The figure shows three views and two pictorial views of one solid part (mm, origin at its lowest corner). Answer the questions. Give positions to 0.01 mm unless a question says otherwise; leave off trailing zeros. Write each loop counter-clockwise with the first axis right and the second up, starting at its lowest first coordinate (ties: lowest second). Pieces come first, ordered by that corner, then holes. Notation, with made-up numbers: (43.5, 3.5) -> (51.5, 3.5) arc R37 cw to (51.5, 42.5) -> close; hole circle Ø6 at (-5.5, 17.5). An arc over 180 degrees is marked (long way). Write item = value, one per line. Start each with the question number.
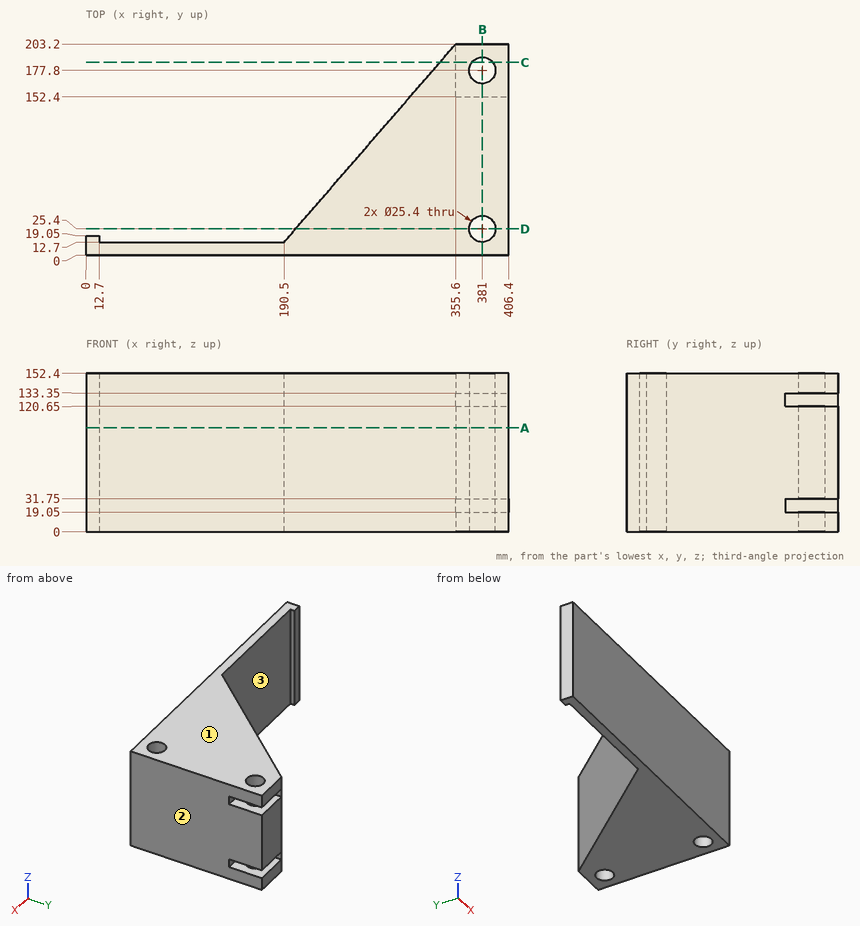
(1) A cutting plane is placed at A-A, the plane z = 100. Write down the section's boundary in (x, y).
(2) Find the intervals of material crossed by line 1 along Y through (x, z) = (380, 44); line 2 along X through (y, z) = (177, 148); line 3 along Y through (x, z) = (20.5, 17), in increasing order.
(3) A cutting plane is placed at D-D, the plane y = 25.4. Write down the section's boundary in (x, z), then the cut area to 3 significant figures.
(4) A cutting plane is placed at B-B, the plane x = 381. Write down the section's boundary in (y, z).
(5) Determine the mould class of the marked faces 1, 2 and 3 for opening direction X: pulls with the +X half, pulls with the -X half, needs draft (parallel to the pull), parting line crosses it, or undercut.
(6) Each of these flat-tipped pins is pushed along its axis until it touches: pin 1 (14 mm diameter, centred on y = 178.5, z = 24, fed in from +X); pin 2 (1 mm diameter, centred on y = 169, z = 124.5, fed in from -X); pin 3 (6.5 mm diameter, centred on x = 4, z = 80, fed in from +Y); pin 4 (1.5 mm diameter, centred on x = 211.5, z = 77, fed in from +Y). Where does it stop, or does it pass through?
(7) A cutting plane is placed at C-C, the plane y = 185.5. Write down the section's boundary in (x, z), then the cut area to 3 significant figures.
Results list:
q1.outline = (0, 0) -> (406.4, 0) -> (406.4, 203.2) -> (355.6, 203.2) -> (190.5, 12.7) -> (12.7, 12.7) -> (12.7, 19.05) -> (0, 19.05) -> close; hole circle Ø25.4 at (381, 25.4); hole circle Ø25.4 at (381, 177.8)
q2.line_1 = 0 to 12.74, 38.06 to 165.14, 190.46 to 203.2
q2.line_2 = 332.89 to 368.33, 393.67 to 406.4
q2.line_3 = 0 to 12.7
q3.outline = (201.51, 0) -> (368.3, 0) -> (368.3, 152.4) -> (201.51, 152.4) -> close; (393.7, 0) -> (406.4, 0) -> (406.4, 152.4) -> (393.7, 152.4) -> close
q3.area = 27,400 mm²
q4.outline = (0, 0) -> (12.7, 0) -> (12.7, 152.4) -> (0, 152.4) -> close; (38.1, 0) -> (165.1, 0) -> (165.1, 19.05) -> (152.4, 19.05) -> (152.4, 31.75) -> (165.1, 31.75) -> (165.1, 120.65) -> (152.4, 120.65) -> (152.4, 133.35) -> (165.1, 133.35) -> (165.1, 152.4) -> (38.1, 152.4) -> close; (190.5, 0) -> (203.2, 0) -> (203.2, 19.05) -> (190.5, 19.05) -> close; (190.5, 31.75) -> (203.2, 31.75) -> (203.2, 120.65) -> (190.5, 120.65) -> close; (190.5, 133.35) -> (203.2, 133.35) -> (203.2, 152.4) -> (190.5, 152.4) -> close
q5.face_1 = needs draft
q5.face_2 = pulls with the +X half
q5.face_3 = undercut
q6.pin_1 = 406.4
q6.pin_2 = 325.53
q6.pin_3 = 19.05
q6.pin_4 = 37.8
q7.outline = (340.26, 0) -> (370.9, 0) -> (370.9, 19.05) -> (355.6, 19.05) -> (355.6, 31.75) -> (370.9, 31.75) -> (370.9, 120.65) -> (355.6, 120.65) -> (355.6, 133.35) -> (370.9, 133.35) -> (370.9, 152.4) -> (340.26, 152.4) -> close; (391.1, 0) -> (406.4, 0) -> (406.4, 19.05) -> (391.1, 19.05) -> close; (391.1, 31.75) -> (406.4, 31.75) -> (406.4, 120.65) -> (391.1, 120.65) -> close; (391.1, 133.35) -> (406.4, 133.35) -> (406.4, 152.4) -> (391.1, 152.4) -> close
q7.area = 6,220 mm²
